from build123d import *

# Parameters (mm, degrees)
CROQUIS1_R              = 20
SALIENTE_EXTRUIR1_DEPTH = 8
CORTAR_EXTRUIR1_DEPTH   = 8
CORTAR_EXTRUIR2_DEPTH   = 10
CROQUIS4_R              = 10
CROQUIS4_R_2            = 2.15
SALIENTE_EXTRUIR2_DEPTH = 3
REDONDEO1_R             = 10
REDONDEO2_R             = 10
CROQUIS5_R              = 2.95
CORTAR_EXTRUIR4_DEPTH   = 31.099222036
REDONDEO4_R             = 1.5


with BuildPart() as part:
    # Croquis1 → Saliente-Extruir1 (new body)
    with BuildSketch(Plane.XY):
        Circle(CROQUIS1_R)
        with BuildLine():
            Line((-1.204159458, 1.2), (1.204159458, 1.2))
            ThreePointArc((1.204159458, 1.2), (0, -1.7), (-1.204159458, 1.2))
        make_face(mode=Mode.SUBTRACT)
    extrude(amount=-SALIENTE_EXTRUIR1_DEPTH)

    # Croquis2 → Cortar-Extruir1 (cut)
    with BuildSketch(Plane.XY):
        with BuildLine():
            ThreePointArc((2.743493279, 19.8109375), (0, 20), (-2.743493279, 19.8109375))
            ThreePointArc((-2.743493279, 19.8109375), (0, 17.25), (2.743493279, 19.8109375))
        make_face()
        with BuildLine():
            ThreePointArc((-15.948597043, 12.068233192), (-12.197270604, 12.196913347), (-12.068700327, 15.948243553))
            ThreePointArc((-12.068700327, 15.948243553), (-14.142342736, 14.141928508), (-15.948597043, 12.068233192))
        make_face()
        with BuildLine():
            ThreePointArc((15.948184756, 12.068778024), (14.141928523, 14.142342722), (12.068310924, 15.948538223))
            ThreePointArc((12.068310924, 15.948538223), (12.197913345, 12.198270606), (15.948184756, 12.068778024))
        make_face()
        with BuildLine():
            ThreePointArc((-19.810790862, -2.744551953), (-17.249000003, -0.000862493), (-19.811065232, 2.742570761))
            ThreePointArc((-19.811065232, 2.742570761), (-19.999999975, -0.00100005), (-19.810790862, -2.744551953))
        make_face()
        with BuildLine():
            ThreePointArc((19.811084118, -2.742434336), (19.999999975, 0.00099995), (19.810809789, 2.744415332))
            ThreePointArc((19.810809789, 2.744415332), (17.251000003, 0.000862507), (19.811084118, -2.742434336))
        make_face()
        with BuildLine():
            ThreePointArc((-12.06710539, -15.949450383), (-12.196050859, -12.198133106), (-15.947390094, -12.069828051))
            ThreePointArc((-15.947390094, -12.069828051), (-14.140928423, -14.143342722), (-12.06710539, -15.949450383))
        make_face()
        with BuildLine():
            ThreePointArc((12.069905665, -15.947331352), (14.143342636, -14.140928508), (15.949391508, -12.067183206))
            ThreePointArc((15.949391508, -12.067183206), (12.199133118, -12.197050847), (12.069905665, -15.947331352))
        make_face()
        with BuildLine():
            ThreePointArc((2.745474352, -19.810663053), (0.001725, -17.250000014), (-2.741512165, -19.811211751))
            ThreePointArc((-2.741512165, -19.811211751), (0.002, -19.9999999), (2.745474352, -19.810663053))
        make_face()
    extrude(amount=-CORTAR_EXTRUIR1_DEPTH, mode=Mode.SUBTRACT)

    # Croquis3 → Cortar-Extruir2 (cut)
    with BuildSketch(Plane(origin=(0, 0, -8), x_dir=(-1, 0, 0), z_dir=(0, 0, -1))):
        Polygon((7.159143338, 0), (3.579571669, 6.2), (-3.579571669, 6.2), (-7.159143338, 0), (-3.579571669, -6.2), (3.579571669, -6.2), align=None)
    extrude(amount=-CORTAR_EXTRUIR2_DEPTH, mode=Mode.SUBTRACT)

    # Croquis4 → Saliente-Extruir2 (add)
    with BuildSketch(Plane(origin=(0, 0, -8), x_dir=(-1, 0, 0), z_dir=(0, 0, -1))):
        with Locations(Location((0, 0, 0), (0, 0, 180))):
            Circle(CROQUIS4_R)
        Circle(CROQUIS4_R_2, mode=Mode.SUBTRACT)
    extrude(amount=SALIENTE_EXTRUIR2_DEPTH)

    # Redondeo1
    # the kernel refuses this fillet: 10 mm, written as the material it adds along each edge
    with BuildSketch(Plane(origin=(0, 0, -8), x_dir=(1, 0, 0), z_dir=(0, 1, 0))) as redondeo1_piece_1:
        with BuildLine():
            CenterArc((17.141428429, 10), REDONDEO1_R, 224.427004001, 45.572995999)
            Line((10, 3), (9.857171431, 2.86))
            ThreePointArc((9.857171431, 2.86), (9.8, 1.5), (9.8, 0))
            Line((9.8, 0), (10, -0.2))
            Line((10, -0.2), (17.141428429, -0.2))
            Line((17.141428429, -0.2), (17.141428429, 0))
        make_face()
    revolve(axis=Axis((0, 0, -8), (0, 0, -1)))

    # Redondeo2
    redondeo2_edges = [part.edges().sort_by_distance(p)[0] for p in [
        (-10, 0, -11),
    ]]
    fillet(redondeo2_edges, radius=REDONDEO2_R)

    # Croquis5 → Cortar-Extruir4 (cut, through all)
    with BuildSketch(Plane.XY):
        with Locations((0, 20)):
            Circle(CROQUIS5_R)
        with Locations((14.142135624, 14.142135624)):
            Circle(CROQUIS5_R)
        with Locations((20, 0)):
            Circle(CROQUIS5_R)
        with Locations((14.142135624, -14.142135624)):
            Circle(CROQUIS5_R)
        with Locations((0, -20)):
            Circle(CROQUIS5_R)
        with Locations((-14.142135624, -14.142135624)):
            Circle(CROQUIS5_R)
        with Locations((-20, 0)):
            Circle(CROQUIS5_R)
        with Locations((-14.142135624, 14.142135624)):
            Circle(CROQUIS5_R)
    extrude(amount=-CORTAR_EXTRUIR4_DEPTH, mode=Mode.SUBTRACT)

    # Redondeo4
    redondeo4_edges = [part.edges().sort_by_distance(p)[0] for p in [
        (-11.908011282, 16.068580127, -4),
        (-16.068580127, 11.908011282, -4),
        (-19.7824375, -2.941966444, -4),
        (-19.7824375, 2.941966444, -4),
        (-16.068580127, -11.908011282, -4),
        (-11.908011282, -16.068580127, -4),
        (2.941966444, -19.7824375, -4),
        (-2.941966444, -19.7824375, -4),
        (11.908011282, -16.068580127, -4),
        (16.068580127, -11.908011282, -4),
        (19.7824375, 2.941966444, -4),
        (19.7824375, -2.941966444, -4),
        (11.908011282, 16.068580127, -4),
        (16.068580127, 11.908011282, -4),
        (-2.941966444, 19.7824375, -4),
        (2.941966444, 19.7824375, -4),
    ]]
    fillet(redondeo4_edges, radius=REDONDEO4_R)


solid = part.part
Can you work these out from the model? Positions are in its coordinate system, mm. A direction names the side the tool comes from. Round coordinates to 2 decimals unless told otherwise and drop trailing zeros. Answer in a Markdown table with one row per item.
(1) Which directions (+Z, -Z, +X, -X, +Y, -Y) give clear straight access to the entire face, cutting with the end or side of a thin tool? Please do faces 1 (the face through (0, -6.2, -4)), 2 (the face through (17, 7, -8)), 3 (the face through (17, -7, -8)).
From the geometry:
| item | result |
|---|---|
| face 1 | +Z |
| face 2 | -Z, +X, +Y |
| face 3 | -Z, +X, -Y |
(2) If we mould it in two halves opening along Y, with no side actions, what happens to faces 4 (the face through (7.6, -18.5, -3.9)), 5 (the face through (7.7, 18.46, -3.94)), 6 (the face through (-12.089, 12.024, -3.944))? For each: released by +Y, released by -Y, zero draft, split by the parting line, or undercut.
From the geometry:
| item | result |
|---|---|
| face 4 | released by -Y |
| face 5 | released by +Y |
| face 6 | undercut |
(3) Please list where these lines run through material, in increasing order: L1, parallel to Y at x = 0, z = -9.1; L2, parallel to Y at x = -7, z = -7.75 (3 decimals); L3, parallel to Z at x = -5.5, y = -7. Write a range as from..to.
From the geometry:
| item | result |
|---|---|
| L1 | y = -12.58..-2.15, 2.15..12.58 |
| L2 | y = -18.735..-0.276, 0.276..18.735 |
| L3 | z = -10.73..0 |
(4) For P1, Ø6, axis at y = -12, z = -3.5, coming from the +X side; P2, Ø3.5, axis at x = 8, y = -15, coming from the -Z side; P3, Ø2, axis at x = -5, y = 17.5, coming from the -Z side; P4, Ø2.5, axis at x = 0, y = 0, coming from the -Z side, each with a flat end and sliding along its axis, tell me the tip position at first contact or that it passes through.
From the geometry:
| item | result |
|---|---|
| P1 | stops at x = 17.86 |
| P2 | stops at z = -8.18 |
| P3 | stops at z = -8 |
| P4 | passes through |
